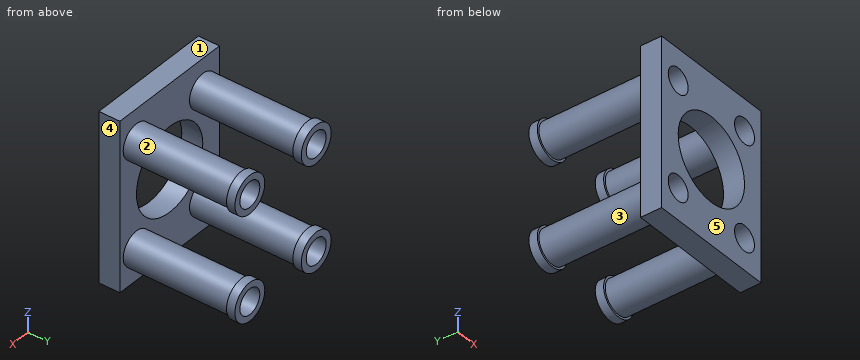
```python
from build123d import *

# Parameters (mm, degrees)
SKETCH1_W           = 38.1
SKETCH1_H           = 50.8
BOSS_EXTRUDE1_DEPTH = 6.35
SKETCH2_R           = 5.08
BOSS_EXTRUDE2_DEPTH = 31.75
SKETCH5_R           = 12.7
CUT_EXTRUDE1_DEPTH  = 45.901280605
SKETCH6_R           = 3.81
CUT_EXTRUDE2_DEPTH  = 50.595085442
BOSS_EXTRUDE3_START = 2.54
SKETCH7_R           = 5.715
SKETCH7_R_2         = 3.81
BOSS_EXTRUDE3_DEPTH = 2.54


with BuildPart() as part:
    # Sketch1 → Boss-Extrude1 (new body)
    with BuildSketch(Plane(origin=(0, 0, 0), x_dir=(1, 0, 0), z_dir=(0, 1, 0))):
        Rectangle(SKETCH1_W, SKETCH1_H)
    extrude(amount=BOSS_EXTRUDE1_DEPTH)

    # Sketch2 → Boss-Extrude2 (add)
    with BuildSketch(Plane(origin=(0, 6.35, 0), x_dir=(1, 0, 0), z_dir=(0, 1, 0))):
        with Locations(Location((-12.7, 15.875, 0), (0, 0, 270))):
            Circle(SKETCH2_R)
        with Locations(Location((12.7, 15.875, 0), (0, 0, 270))):
            Circle(SKETCH2_R)
        with Locations(Location((12.7, -15.875, 0), (0, 0, 270))):
            Circle(SKETCH2_R)
        with Locations(Location((-12.7, -15.875, 0), (0, 0, 270))):
            Circle(SKETCH2_R)
    extrude(amount=BOSS_EXTRUDE2_DEPTH)

    # Sketch5 → Cut-Extrude1 (cut, through all)
    with BuildSketch(Plane(origin=(0, 6.35, 0), x_dir=(1, 0, 0), z_dir=(0, 1, 0))):
        with Locations(Location((0, 0, 0), (0, 0, 270))):
            Circle(SKETCH5_R)
    extrude(amount=-CUT_EXTRUDE1_DEPTH, mode=Mode.SUBTRACT)

    # Sketch6 → Cut-Extrude2 (cut, through all)
    with BuildSketch(Plane(origin=(0, 38.1, 0), x_dir=(1, 0, 0), z_dir=(0, 1, 0))):
        with Locations(Location((-12.7, 15.875, 0), (0, 0, 270))):
            Circle(SKETCH6_R)
        with Locations(Location((12.7, 15.875, 0), (0, 0, 270))):
            Circle(SKETCH6_R)
        with Locations(Location((12.7, -15.875, 0), (0, 0, 270))):
            Circle(SKETCH6_R)
        with Locations(Location((-12.7, -15.875, 0), (0, 0, 270))):
            Circle(SKETCH6_R)
    extrude(amount=-CUT_EXTRUDE2_DEPTH, mode=Mode.SUBTRACT)

    # Sketch7 → Boss-Extrude3 (add)
    # profile 1 of 4: a face of its own
    with BuildSketch(Plane(origin=(0, 38.1, 0), x_dir=(1, 0, 0), z_dir=(0, 1, 0)).offset(BOSS_EXTRUDE3_START)):
        with Locations(Location((-12.7, 15.875, 0), (0, 0, 270))):
            Circle(SKETCH7_R)
        with Locations(Location((-12.7, 15.875, 0), (0, 0, 270))):
            Circle(SKETCH7_R_2, mode=Mode.SUBTRACT)
    # profile 2 of 4: a face of its own
    with BuildSketch(Plane(origin=(0, 38.1, 0), x_dir=(1, 0, 0), z_dir=(0, 1, 0)).offset(BOSS_EXTRUDE3_START)):
        with Locations(Location((-12.7, -15.875, 0), (0, 0, 270))):
            Circle(SKETCH7_R)
        with Locations(Location((-12.7, -15.875, 0), (0, 0, 270))):
            Circle(SKETCH7_R_2, mode=Mode.SUBTRACT)
    # profile 3 of 4: a face of its own
    with BuildSketch(Plane(origin=(0, 38.1, 0), x_dir=(1, 0, 0), z_dir=(0, 1, 0)).offset(BOSS_EXTRUDE3_START)):
        with Locations(Location((12.7, -15.875, 0), (0, 0, 270))):
            Circle(SKETCH7_R)
        with Locations(Location((12.7, -15.875, 0), (0, 0, 270))):
            Circle(SKETCH7_R_2, mode=Mode.SUBTRACT)
    # profile 4 of 4: a face of its own
    with BuildSketch(Plane(origin=(0, 38.1, 0), x_dir=(1, 0, 0), z_dir=(0, 1, 0)).offset(BOSS_EXTRUDE3_START)):
        with Locations(Location((12.7, 15.875, 0), (0, 0, 270))):
            Circle(SKETCH7_R)
        with Locations(Location((12.7, 15.875, 0), (0, 0, 270))):
            Circle(SKETCH7_R_2, mode=Mode.SUBTRACT)
    extrude(amount=-BOSS_EXTRUDE3_DEPTH)


solid = part.part
```
Input: part model. Units: mm. Frame: model coordinates. Face numbers are marked on the shaded views. A direction names the side the tool comes from. Coordinates: 2 decimals unless noted, no trailing zeros. Loops run counter-clockwise (first coordinate to the right, second up) from the corner with the lowest first, then second, coordinate; pieces in that order, holes last. Notation, with made-up numbers: M 51,77.25 L 60,77.25 A21 cw 60,111.25 Z; hole C -27.5,25.5 d8. An arc over 180 degrees is marked long. Use a Markdown table: item, result. Add a question column.
1) Draft query along Y for the marked faces 3, 4 and 5. Return one class per face: +Y half, -Y half, draft (parallel to the pull), parting line (faces both ways), or undercut.
2) Line query: L1, parallel to X at y = 13.5, z = -16; L2, parallel to Z at x = -15.5, y = 7; L3, parallel to Z at x = -12, y = 29. Output: solid intervals per line, ascending. Write a range as from..to.
3) Section C-C, the plane y = 5. Return the cut outline in (x, z) (3 decimals).
4) Section A-A, the plane y = 29. Return the cut outline in (x, z) (3 decimals), plus the area to 3 significant figures.
5) Set-up query: the marked faces 1 and 2. Return all of +Z, -Z, +X, -X, +Y, -Y with unobstructed straight access to the full face (end or side cutting, diameter ignored); none if empty.
6) Pin query (flat end, axial travel): P1, Ø2, axis at y = 32.5, z = -11, coming from the +X side; P2, Ø2, axis at x = -10.5, z = -6.5, coming from the -Y side; P3, Ø11.5, axis at x = 3.5, z = 4, coming from the +Y side; P4, Ø5, axis at x = 7.5, y = 31, coming from the +Z side. Return the tip coordinate at first contact, or that it passes through.
7) Section D-D, the plane z = 0. Return the cut outline in (x, y), plus the area to 3 significant figures.
8) Section B-B, the plane x = 0. Return the cut outline in (y, z).
Answer below:
| question | item | result |
|---|---|---|
| 1 | face 3 | undercut |
| 1 | face 4 | draft |
| 1 | face 5 | -Y half |
| 2 | L1 | -17.78..-16.51, -8.89..-7.62, 7.62..8.89, 16.51..17.78 |
| 2 | L2 | -20.11..-18.46, -13.29..-11.64, 11.64..13.29, 18.46..20.11 |
| 2 | L3 | -20.91..-19.62, -12.13..-10.84, 10.84..12.13, 19.62..20.91 |
| 3 | outline | M -19.05,-25.4 L 19.05,-25.4 L 19.05,25.4 L -19.05,25.4 Z; hole C -12.7,-15.875 d7.62; hole C -12.7,15.875 d7.62; hole C 0,0 d25.4; hole C 12.7,-15.875 d7.62; hole C 12.7,15.875 d7.62 |
| 4 | outline | C -12.7,-15.875 d10.16; C -12.7,15.875 d10.16; C 12.7,-15.875 d10.16; C 12.7,15.875 d10.16; hole C -12.7,-15.875 d7.62; hole C -12.7,15.875 d7.62; hole C 12.7,-15.875 d7.62; hole C 12.7,15.875 d7.62 |
| 4 | area | 142 mm2 |
| 5 | face 1 | +Z, +X, -X, +Y, -Y |
| 5 | face 2 | none |
| 6 | P1 | x = 15.98 |
| 6 | P2 | y = 0 |
| 6 | P3 | through |
| 6 | P4 | z = 20.18 |
| 7 | outline | M -19.05,0 L -12.7,0 L -12.7,6.35 L -19.05,6.35 Z; M 12.7,0 L 19.05,0 L 19.05,6.35 L 12.7,6.35 Z |
| 7 | area | 80.6 mm2 |
| 8 | outline | M 0,-25.4 L 6.35,-25.4 L 6.35,-12.7 L 0,-12.7 Z; M 0,12.7 L 6.35,12.7 L 6.35,25.4 L 0,25.4 Z |
